from build123d import *

# Parameters (mm, degrees)
BOSS_EXTRUDE1_DEPTH = 10
SKETCH10_W          = 70
SKETCH10_H          = 80
BOSS_EXTRUDE6_DEPTH = 78
CUT_EXTRUDE7_DEPTH  = 46
SKETCH15_R          = 1.25
BOSS_EXTRUDE7_DEPTH = 4
SKETCH17_R          = 2.25
CUT_EXTRUDE9_DEPTH  = 2.5
SKETCH19_W          = 72
SKETCH19_H          = 76
CUT_EXTRUDE11_DEPTH = 70
SKETCH20_R          = 1.65
CUT_EXTRUDE12_DEPTH = 10
SKETCH21_R          = 12.5
CUT_EXTRUDE13_DEPTH = 10
CUT_EXTRUDE14_DEPTH = 3
FILLET3_R           = 5
SKETCH23_W          = 2
SKETCH23_H          = 4.2
CUT_EXTRUDE15_DEPTH = 4
SKETCH24_R          = 1.15
CUT_EXTRUDE16_DEPTH = 118
SKETCH27_W          = 4.2
SKETCH27_H          = 2
CUT_EXTRUDE17_DEPTH = 4
SKETCH28_R          = 1.15
CUT_EXTRUDE18_DEPTH = 121.187353744
FILLET4_R           = 35
SKETCH29_R          = 14.814456412
CUT_EXTRUDE19_DEPTH = 4


with BuildPart() as part:
    # Sketch1 → Boss-Extrude1 (new body)
    with BuildSketch(Plane.XY):
        with BuildLine():
            Line((-20, -35), (20, -35))
            ThreePointArc((20, -35), (27.071067812, -32.071067812), (30, -25))
            Line((30, -25), (30, 25))
            ThreePointArc((30, 25), (27.071067812, 32.071067812), (20, 35))
            Line((20, 35), (-20, 35))
            ThreePointArc((-20, 35), (-27.071067812, 32.071067812), (-30, 25))
            Line((-30, 25), (-30, -25))
            ThreePointArc((-30, -25), (-27.071067812, -32.071067812), (-20, -35))
        make_face()
    extrude(amount=-BOSS_EXTRUDE1_DEPTH)

    # Sketch10 → Boss-Extrude6 (add)
    with BuildSketch(Plane(origin=(0, 0, -10), x_dir=(-1, 0, 0), z_dir=(0, 0, -1))):
        with Locations((0, -3)):
            Rectangle(SKETCH10_W, SKETCH10_H)
    extrude(amount=BOSS_EXTRUDE6_DEPTH)

    # Sketch14 → Cut-Extrude7 (cut)
    with BuildSketch(Plane.XY):
        with BuildLine():
            Line((20, 31), (-20, 31))
            ThreePointArc((-20, 31), (-24.242640687, 29.242640687), (-26, 25))
            Line((-26, 25), (-26, -25))
            ThreePointArc((-26, -25), (-24.242640687, -29.242640687), (-20, -31))
            Line((-20, -31), (20, -31))
            ThreePointArc((20, -31), (24.242640687, -29.242640687), (26, -25))
            Line((26, -25), (26, 25))
            ThreePointArc((26, 25), (24.242640687, 29.242640687), (20, 31))
        make_face()
    extrude(amount=-CUT_EXTRUDE7_DEPTH, mode=Mode.SUBTRACT)

    # Sketch15 → Boss-Extrude7 (add)
    with BuildSketch(Plane.XY):
        with BuildLine():
            Line((-20, 31), (-10.65, 31))
            Line((-10.65, 31), (-10.65, -26))
            Line((-10.65, -26), (10.65, -26))
            Line((10.65, -26), (10.65, 31))
            Line((10.65, 31), (20, 31))
            ThreePointArc((20, 31), (24.242640687, 29.242640687), (26, 25))
            Line((26, 25), (26, -25))
            ThreePointArc((26, -25), (24.242640687, -29.242640687), (20, -31))
            Line((20, -31), (-20, -31))
            ThreePointArc((-20, -31), (-24.242640687, -29.242640687), (-26, -25))
            Line((-26, -25), (-26, 25))
            ThreePointArc((-26, 25), (-24.242640687, 29.242640687), (-20, 31))
        make_face()
        with Locations((13.5, -7)):
            Circle(SKETCH15_R, mode=Mode.SUBTRACT)
        with Locations((13.5, -15)):
            Circle(SKETCH15_R, mode=Mode.SUBTRACT)
        with Locations((13.5, -23)):
            Circle(SKETCH15_R, mode=Mode.SUBTRACT)
        with Locations(Location((-13.5, -7, 0), (0, 0, 180))):
            Circle(SKETCH15_R, mode=Mode.SUBTRACT)
        with Locations(Location((-13.5, -15, 0), (0, 0, 180))):
            Circle(SKETCH15_R, mode=Mode.SUBTRACT)
        with Locations(Location((-13.5, -23, 0), (0, 0, 180))):
            Circle(SKETCH15_R, mode=Mode.SUBTRACT)
    extrude(amount=-BOSS_EXTRUDE7_DEPTH)

    # Sketch17 → Cut-Extrude9 (cut)
    with BuildSketch(Plane.XY):
        with Locations((-13.5, -7)):
            Circle(SKETCH17_R)
        with Locations((-13.5, -15)):
            Circle(SKETCH17_R)
        with Locations((-13.5, -23)):
            Circle(SKETCH17_R)
        with Locations((13.5, -7)):
            Circle(SKETCH17_R)
        with Locations((13.5, -15)):
            Circle(SKETCH17_R)
        with Locations((13.5, -23)):
            Circle(SKETCH17_R)
    extrude(amount=-CUT_EXTRUDE9_DEPTH, mode=Mode.SUBTRACT)

    # Sketch19 → Cut-Extrude11 (cut)
    with BuildSketch(Plane(origin=(35, 0, 0), x_dir=(0, 0, -1), z_dir=(1, 0, 0))):
        with Locations((52, -1)):
            Rectangle(SKETCH19_W, SKETCH19_H)
    extrude(amount=-CUT_EXTRUDE11_DEPTH, mode=Mode.SUBTRACT)

    # Sketch20 → Cut-Extrude12 (cut)
    with BuildSketch(Plane.XZ.offset(43)):
        with Locations(Location((28, -52, 0), (0, 0, 270))):
            Circle(SKETCH20_R)
        with Locations(Location((0, -80, 0), (0, 0, 270))):
            Circle(SKETCH20_R)
        with Locations(Location((-28, -52, 0), (0, 0, 270))):
            Circle(SKETCH20_R)
    extrude(amount=-CUT_EXTRUDE12_DEPTH, mode=Mode.SUBTRACT)

    # Sketch21 → Cut-Extrude13 (cut)
    with BuildSketch(Plane(origin=(0, -39, 0), x_dir=(1, 0, 0), z_dir=(0, 1, 0))):
        with Locations(Location((0, 52, 0), (0, 0, 270))):
            Circle(SKETCH21_R)
    extrude(amount=-CUT_EXTRUDE13_DEPTH, mode=Mode.SUBTRACT)

    # Sketch22 → Cut-Extrude14 (cut)
    with BuildSketch(Plane(origin=(0, -39, 0), x_dir=(1, 0, 0), z_dir=(0, 1, 0))):
        Polygon((0, 83.233161507), (-2.8, 81.616580754), (-2.8, 78.383419246), (0, 76.766838493), (2.8, 78.383419246), (2.8, 81.616580754), align=None)
        Polygon((-30.8, 50.383419246), (-28, 48.766838493), (-25.2, 50.383419246), (-25.2, 53.616580754), (-28, 55.233161507), (-30.8, 53.616580754), align=None)
        Polygon((28, 55.233161507), (25.2, 53.616580754), (25.2, 50.383419246), (28, 48.766838493), (30.8, 50.383419246), (30.8, 53.616580754), align=None)
    extrude(amount=-CUT_EXTRUDE14_DEPTH, mode=Mode.SUBTRACT)

    # Fillet3
    fillet3_edges = [part.edges().sort_by_distance(p)[0] for p in [
        (0, -39, -16),
        (0, -43, -10),
    ]]
    fillet(fillet3_edges, radius=FILLET3_R)

    # Sketch23 → Cut-Extrude15 (cut)
    with BuildSketch(Plane(origin=(0, 0, -16), x_dir=(-1, 0, 0), z_dir=(0, 0, -1))):
        with Locations((-30, -30.9)):
            Rectangle(SKETCH23_W, SKETCH23_H)
    cut_extrude15 = extrude(amount=-CUT_EXTRUDE15_DEPTH, mode=Mode.SUBTRACT)

    # Sketch24 → Cut-Extrude16 (cut, through all)
    with BuildSketch(Plane(origin=(29, 0, 0), x_dir=(0, 0, -1), z_dir=(1, 0, 0))):
        with Locations(Location((14, -30.9, 0), (0, 0, 90))):
            Circle(SKETCH24_R)
    cut_extrude16 = extrude(amount=CUT_EXTRUDE16_DEPTH, mode=Mode.SUBTRACT)

    # Mirror1: Cut-Extrude15, Cut-Extrude16 across plane
    add(cut_extrude15.mirror(Plane(origin=(0, 0, 0), x_dir=(0, 0, 1), z_dir=(1, 0, 0))), mode=Mode.SUBTRACT)
    add(cut_extrude16.mirror(Plane(origin=(0, 0, 0), x_dir=(0, 0, 1), z_dir=(1, 0, 0))), mode=Mode.SUBTRACT)

    # Sketch27 → Cut-Extrude17 (cut)
    with BuildSketch(Plane(origin=(0, 0, -16), x_dir=(-1, 0, 0), z_dir=(0, 0, -1))):
        with Locations((27.9, 32)):
            Rectangle(SKETCH27_W, SKETCH27_H)
        with Locations((-27.9, 32)):
            Rectangle(SKETCH27_W, SKETCH27_H)
    extrude(amount=-CUT_EXTRUDE17_DEPTH, mode=Mode.SUBTRACT)

    # Sketch28 → Cut-Extrude18 (cut, through all)
    with BuildSketch(Plane(origin=(0, 31, 0), x_dir=(1, 0, 0), z_dir=(0, 1, 0))):
        with Locations(Location((-27.9, 14, 0), (0, 0, 180))):
            Circle(SKETCH28_R)
    cut_extrude18 = extrude(amount=CUT_EXTRUDE18_DEPTH, mode=Mode.SUBTRACT)

    # Mirror2: Cut-Extrude18 across plane
    add(cut_extrude18.mirror(Plane(origin=(0, 0, 0), x_dir=(0, 0, 1), z_dir=(1, 0, 0))), mode=Mode.SUBTRACT)

    # Fillet4
    fillet4_edges = [part.edges().sort_by_distance(p)[0] for p in [
        (35, -41, -88),
        (-35, -41, -88),
    ]]
    fillet(fillet4_edges, radius=FILLET4_R - 0.0001)  # a hair under: the kernel refuses the full size

    # Sketch29 → Cut-Extrude19 (cut)
    with BuildSketch(Plane.XY):
        with Locations((0, 6.918633542)):
            Circle(SKETCH29_R)
    extrude(amount=-CUT_EXTRUDE19_DEPTH, mode=Mode.SUBTRACT)


solid = part.part
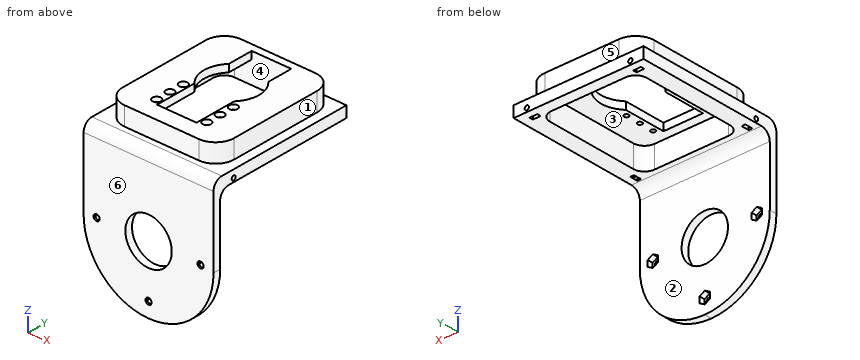
Check sheet for the modelled part. Datum: model origin and axes. Units: mm. Face numbers are marked on the shaded views. A direction names the side the tool comes from. Give positions to 0.01 mm unless a question says otherwise; leave off trailing zeros. Loops run counter-clockwise (first coordinate to the right, second up) from the corner with the lowest first, then second, coordinate; pieces in that order, holes last. Notation, with made-up numbers: M -24,9 L 10,9 A16 ccw 10,36 Z; hole C 77,53 d6. An arc over 180 degrees is marked long. Answer as a JSON object with one key per item and string values. Group by question number.
Q1. Material ranges on line 1 along Y through (x, z) = (13.5, -3); line 2 along Z through (x, y) = (33, -30); line 3 along Y through (x, z) = (-14.5, -15.5), recorded low to high. Write a range as [from, to].
Q2. Cross-section at D-D on x = 8.5. Record the cut outline in (y, z).
Q3. Cross-section at A-A on y = -15. Give the number of separate pieces and of enclosed holes in the cut face, then the cut area to 3 significant figures.
Q4. Access from +Z, -Z, +X, -X, +Y, -Y to the whole of each face (thin tool, end or side, straight path). Record for the marked faces 1, 2 and 3.
Q5. Go/stop test with flat-tipped pins: P1, Ø1.5, axis at x = -21.5, y = 7, coming from the +Z side; P2, Ø2, axis at x = 3.5, z = -34, coming from the +Y side; P3, Ø4.5, axis at y = -17.5, z = -3, coming from the +X side; P4, Ø5, axis at y = 5.5, z = -6, coming from the -X side. Record where each tip stops, or that it passes through.
Q6. Cross-section at C-C on z = -61.5. Record the cut outline in (x, y), then the cut area to 3 significant figures.
Q7. Cross-section at B-B on y = 21. Record the cut outline in (x, z).
Q8. Release check for a two-part mould opening along Y. For the marked faces 4, 5 and 6 record: released by +Y, released by -Y, zero draft, split by the parting line, or undercut.
Evaluation:
{
 "1": {"line 1": "y = [-35, -24.25], [-21.75, -16.25], [-13.75, -8.25], [-5.75, 0.82], [13.02, 35]", "line 2": "z = [-16, -14.72], [-13.28, -10]", "line 3": "y = [-43, -31], [31, 37]"},
 "2": {"outline": "M -43,-86.95 L -39,-86.95 L -39,-61.17 L -43,-61.17 Z; M -43,-42.83 L -39,-42.83 L -39,-21 A5 cw -34,-16 L -31,-16 L -31,-4 L -26,-4 L -26,0 L -35,0 L -35,-10 L -38,-10 A5 ccw -43,-15 Z; M 31,-16 L 37,-16 L 37,-10 L 35,-10 L 35,0 L 31,0 Z"},
 "3": {"separate pieces": "4", "enclosed holes": "0", "area": "281 mm2"},
 "4": {"face 1": "+Z, +X, +Y, -Y", "face 2": "-Z, +X, -X, +Y", "face 3": "-Z"},
 "5": {"P1": "stops at z = 0", "P2": "stops at y = -39", "P3": "stops at x = 30", "P4": "stops at x = -30"},
 "6": {"outline": "M -33.95,-43 L -8.12,-43 L -8.12,-39 L -33.95,-39 Z; M 8.12,-43 L 33.95,-43 L 33.95,-39 L 8.12,-39 Z", "area": "207 mm2"},
 "7": {"outline": "M -35,-16 L -26,-16 L -26,-4 L -10.65,-4 L -10.65,0 L -30,0 L -30,-10 L -35,-10 Z; M 10.65,-4 L 26,-4 L 26,-16 L 35,-16 L 35,-10 L 30,-10 L 30,0 L 10.65,0 Z"},
 "8": {"face 4": "undercut", "face 5": "released by +Y", "face 6": "released by -Y"}
}
